Geometry: final body of the model. Coordinates: model frame, mm. Give positions to 0.01 mm unless a question says otherwise; leave off trailing zeros. Write each loop counter-clockwise with the first axis right and the second up, starting at its lowest first coordinate (ties: lowest second). Pieces come first, ordered by that corner, then holes.
from build123d import *

# Parameters (mm, degrees)
SKETCH1_W               = 671.5125
SKETCH1_H               = 299.466
BOSS_EXTRUDE1_DEPTH     = 0.1016
BOSS_EXTRUDE2_DEPTH     = 0.2032
FILLET1_R               = 25.4
SKETCH3_R               = 17.5
SKETCH3_R_2             = 14.2875
SKETCH3_R_3             = 2.95
CUT_EXTRUDE1_DEPTH      = 1
CUT_EXTRUDE1_DEPTH_BACK = 1.2032
SKETCH4_W               = 671.5125
SKETCH4_H               = 33.0708508
CUT_EXTRUDE2_DEPTH      = 1
CUT_EXTRUDE2_DEPTH_BACK = 1.2032
BOSS_EXTRUDE3_DEPTH     = 0.2032


with BuildPart() as part:
    # Sketch1 → Boss-Extrude1 (new body, symmetric)
    with BuildSketch(Plane(origin=(0, 0, 0), x_dir=(1, 0, 0), z_dir=(0, 1, 0))):
        Rectangle(SKETCH1_W, SKETCH1_H)
    extrude(amount=BOSS_EXTRUDE1_DEPTH, both=True)

    # Sketch2 → Boss-Extrude2 (add)
    with BuildSketch(Plane(origin=(0, 0.1016, 0), x_dir=(1, 0, 0), z_dir=(0, 1, 0))):
        Polygon((335.75625, -149.733), (374.643853371, -149.733), (412.08325, 116.6621492), (335.75625, 116.6621492), align=None)
        Polygon((-335.75625, 116.6621492), (-335.75625, -149.733), (-374.643853371, -149.733), (-412.08325, 116.6621492), align=None)
    extrude(amount=-BOSS_EXTRUDE2_DEPTH)

    # Fillet1
    fillet1_edges = [part.edges().sort_by_distance(p)[0] for p in [
        (374.643853371, 0, 149.733),
        (412.08325, 0, -116.6621492),
        (-412.08325, 0, -116.6621492),
        (-374.643853371, 0, 149.733),
    ]]
    fillet(fillet1_edges, radius=FILLET1_R)

    # Sketch3 → Cut-Extrude1 (cut, two sides)
    with BuildSketch(Plane(origin=(0, 0.1016, 0), x_dir=(1, 0, 0), z_dir=(0, 1, 0))) as cut_extrude1_sk:
        with Locations((-275.836957508, -19.05)):
            Circle(SKETCH3_R)
        with Locations((-180.836957508, 7.95)):
            Circle(SKETCH3_R_2)
        with Locations((-145.836957508, 16.95)):
            Circle(SKETCH3_R_2)
        with Locations((-145.836957508, -19.05)):
            Circle(SKETCH3_R_2)
        with Locations((-180.836957508, -28.05)):
            Circle(SKETCH3_R_2)
        with Locations((-212.086957508, -10.05)):
            Circle(SKETCH3_R_2)
        with Locations((-212.086957508, -46.05)):
            Circle(SKETCH3_R_2)
        with Locations((-212.086957508, 82.55)):
            Circle(SKETCH3_R_2)
        with Locations((-164.36967051, 82.55)):
            Circle(SKETCH3_R_2)
        with Locations((130.563042492, -19.05)):
            Circle(SKETCH3_R)
        with Locations((225.563042492, 7.95)):
            Circle(SKETCH3_R_2)
        with Locations((260.563042492, 16.95)):
            Circle(SKETCH3_R_2)
        with Locations((260.563042492, -19.05)):
            Circle(SKETCH3_R_2)
        with Locations((225.563042492, -28.05)):
            Circle(SKETCH3_R_2)
        with Locations((194.313042492, -10.05)):
            Circle(SKETCH3_R_2)
        with Locations((194.313042492, -46.05)):
            Circle(SKETCH3_R_2)
        with Locations((194.313042492, 82.55)):
            Circle(SKETCH3_R_2)
        with Locations((242.03032949, 82.55)):
            Circle(SKETCH3_R_2)
        with Locations((-308.636957508, 18.9)):
            Circle(SKETCH3_R_3)
        with Locations((-243.036957508, 18.9)):
            Circle(SKETCH3_R_3)
        with Locations((-308.636957508, -57)):
            Circle(SKETCH3_R_3)
        with Locations((-243.036957508, -57)):
            Circle(SKETCH3_R_3)
        with Locations((97.763042492, 18.9)):
            Circle(SKETCH3_R_3)
        with Locations((163.363042492, 18.9)):
            Circle(SKETCH3_R_3)
        with Locations((97.763042492, -57)):
            Circle(SKETCH3_R_3)
        with Locations((163.363042492, -57)):
            Circle(SKETCH3_R_3)
        with Locations((-44.45, 57.15)):
            Circle(SKETCH3_R_2)
        with Locations((0, 57.15)):
            Circle(SKETCH3_R_2)
        with Locations((44.45, 57.15)):
            Circle(SKETCH3_R_2)
    extrude(amount=CUT_EXTRUDE1_DEPTH, mode=Mode.SUBTRACT)
    extrude(cut_extrude1_sk.sketch, amount=-CUT_EXTRUDE1_DEPTH_BACK, mode=Mode.SUBTRACT)

    # Sketch4 → Cut-Extrude2 (cut, two sides)
    with BuildSketch(Plane(origin=(0, 0.1016, 0), x_dir=(1, 0, 0), z_dir=(0, 1, 0))) as cut_extrude2_sk:
        with Locations((0, 133.1975746)):
            Rectangle(SKETCH4_W, SKETCH4_H)
    extrude(amount=CUT_EXTRUDE2_DEPTH, mode=Mode.SUBTRACT)
    extrude(cut_extrude2_sk.sketch, amount=-CUT_EXTRUDE2_DEPTH_BACK, mode=Mode.SUBTRACT)

    # Sketch5 → Boss-Extrude3 (add)
    with BuildSketch(Plane(origin=(0, 0.1016, 0), x_dir=(1, 0, 0), z_dir=(0, 1, 0))):
        with BuildLine():
            Line((382.863892457, 124.9679492), (-382.863892457, 124.9679492))
            ThreePointArc((-382.863892457, 124.9679492), (-408.301982626, 113.375143619), (-416.241669928, 86.571208494))
            Line((-416.241669928, 86.571208494), (-385.941747702, -129.023940706))
            ThreePointArc((-385.941747702, -129.023940706), (-374.67696465, -149.771090169), (-352.56397023, -158.0388))
            Line((-352.56397023, -158.0388), (352.56397023, -158.0388))
            ThreePointArc((352.56397023, -158.0388), (374.67696465, -149.771090169), (385.941747702, -129.023940706))
            Line((385.941747702, -129.023940706), (416.241669928, 86.571208494))
            ThreePointArc((416.241669928, 86.571208494), (408.301982626, 113.375143619), (382.863892457, 124.9679492))
        make_face()
        with BuildLine():
            Line((382.863892457, 116.6621492), (-382.863892457, 116.6621492))
            ThreePointArc((-382.863892457, 116.6621492), (-402.033515794, 107.926048536), (-408.016701403, 87.727152436))
            Line((-408.016701403, 87.727152436), (-377.716779176, -127.867996764))
            ThreePointArc((-377.716779176, -127.867996764), (-369.227869567, -143.502623338), (-352.56397023, -149.733))
            Line((-352.56397023, -149.733), (352.56397023, -149.733))
            ThreePointArc((352.56397023, -149.733), (369.227869567, -143.502623338), (377.716779176, -127.867996764))
            Line((377.716779176, -127.867996764), (408.016701403, 87.727152436))
            ThreePointArc((408.016701403, 87.727152436), (402.033515794, 107.926048536), (382.863892457, 116.6621492))
        make_face(mode=Mode.SUBTRACT)
    extrude(amount=-BOSS_EXTRUDE3_DEPTH)


solid = part.part
Q1. Section B-B on y = 0.05. Count the separate pieces of the cut face and the enclosed holes in it, plus the area to 3 significant figures.
Filled sheet:
separate pieces: 1
enclosed holes: 29
area: 212,000 mm2
Q2. Pin query (flat end, axial travel): P1, Ø23, axis at x = -180.84, z = -7.95, coming from the +Y side. Return the tip coordinate at first contact, or that it passes through.
Filled sheet:
P1: passes through
Q3. Ray query, line 1 along X through (y, z) = (0, -78.5); line 2 along X through (y, z) = (0.05, -28); line 3 along Z through (x, y) = (238, 0.05). Return the intervals inside material, ascending.
Filled sheet:
line 1: x = -415.11 to -225.79, -198.39 to -178.07, -150.67 to 180.61, 208.01 to 228.33, 255.73 to 415.11
line 2: x = -408.01 to -154.89, -136.78 to 251.51, 269.62 to 408.01
line 3: z = -124.97 to -96.26, -68.84 to -14.98, -0.92 to 21.02, 35.08 to 158.04
Q4. Section C-C on z = 118. Output: boundary loops of the cut face in (x, y).
Filled sheet:
outline: (-387.49, -0.1) - (387.49, -0.1) - (387.49, 0.1) - (-387.49, 0.1) - close
Q5. Section A-A on x = 127. Output: boundary loops of the cut face in (y, z).
Filled sheet:
outline: (-0.1, -124.97) - (0.1, -124.97) - (0.1, 1.92) - (-0.1, 1.92) - close; (-0.1, 36.18) - (0.1, 36.18) - (0.1, 158.04) - (-0.1, 158.04) - close
